Can you work these out from the model? Positions are in its coordinate system, mm. Face numbers are marked on the shaded views. A direction names the side the tool comes from. Coordinates: 2 decimals unless noted, no trailing zeros. Loops run counter-clockwise (first coordinate to the right, second up) from the corner with the lowest first, then second, coordinate; pieces in that order, holes last.
```python
from build123d import *

# Parameters (mm, degrees)
CYLINDER013_R     = 9.3
CYLINDER013_DEPTH = 30
BOX004_W          = 38
BOX004_H          = 16
BOX004_DEPTH      = 16
FILLET002_R       = 1
BOX003_W          = 20
BOX003_H          = 33
BOX003_DEPTH      = 16
FILLET001_R       = 1
BOX002_W          = 33
BOX002_H          = 27
BOX002_DEPTH      = 20
FILLET_R          = 2
CHAMFER003_SIZE   = 12
CHAMFER004_SIZE   = 18
CHAMFER005_SIZE   = 6.7
CHAMFER006_SIZE   = 6.8
CYLINDER012_R     = 9.3
CYLINDER012_DEPTH = 30
CYLINDER011_R     = 14
CYLINDER011_DEPTH = 15


with BuildPart() as cilindro013:
    # Cylinder013 → Cylinder013 (new body)
    with BuildSketch(Plane(origin=(27, 199, 74), x_dir=(1, 0, 0), z_dir=(0, -1, 0))):
        Circle(CYLINDER013_R)
    extrude(amount=CYLINDER013_DEPTH)


with BuildPart() as fillet002:
    # Box004 → Box004 (new body)
    with BuildSketch(Plane(origin=(-7, 189, 60), x_dir=(1, 0, 0), z_dir=(0, 0, 1))):
        with Locations((19, 8)):
            Rectangle(BOX004_W, BOX004_H)
    extrude(amount=BOX004_DEPTH)

    # Fillet002
    fillet002_edges = [fillet002.edges().sort_by_distance(p)[0] for p in [
        (12, 189, 60),
    ]]
    fillet(fillet002_edges, radius=FILLET002_R)


with BuildPart() as fillet001:
    # Box003 → Box003 (new body)
    with BuildSketch(Plane(origin=(-7, 172, 60), x_dir=(1, 0, 0), z_dir=(0, 0, 1))):
        with Locations((10, 16.5)):
            Rectangle(BOX003_W, BOX003_H)
    extrude(amount=BOX003_DEPTH)

    # Fillet001
    fillet001_edges = [fillet001.edges().sort_by_distance(p)[0] for p in [
        (13, 188.5, 60),
    ]]
    fillet(fillet001_edges, radius=FILLET001_R)


with BuildPart() as cut006:
    # Box002 → Box002 (new body)
    with BuildSketch(Plane(origin=(-5, 174, 53.3), x_dir=(1, 0, 0), z_dir=(0, 0, 1))):
        with Locations((16.5, 13.5)):
            Rectangle(BOX002_W, BOX002_H)
    extrude(amount=BOX002_DEPTH)

    # Fillet
    fillet_edges = [cut006.edges().sort_by_distance(p)[0] for p in [
        (-5, 201, 63.3),
    ]]
    fillet(fillet_edges, radius=FILLET_R)

    # Chamfer003
    chamfer003_edges = [cut006.edges().sort_by_distance(p)[0] for p in [
        (28, 201, 63.3),
    ]]
    chamfer(chamfer003_edges, length=CHAMFER003_SIZE)

    # Chamfer004
    chamfer004_edges = [cut006.edges().sort_by_distance(p)[0] for p in [
        (-5, 174, 63.3),
    ]]
    chamfer(chamfer004_edges, length=CHAMFER004_SIZE)

    # Chamfer005
    chamfer005_edges = [cut006.edges().sort_by_distance(p)[0] for p in [
        (20.5, 174, 53.3),
    ]]
    chamfer(chamfer005_edges, length=CHAMFER005_SIZE)

    # Chamfer006
    chamfer006_edges = [cut006.edges().sort_by_distance(p)[0] for p in [
        (28, 184.85, 53.3),
    ]]
    chamfer(chamfer006_edges, length=CHAMFER006_SIZE)

    # Cut004: cut Fillet001
    add(fillet001.part, mode=Mode.SUBTRACT)

    # Cut005: cut Fillet002
    add(fillet002.part, mode=Mode.SUBTRACT)

    # Cut006: cut Cilindro013
    add(cilindro013.part, mode=Mode.SUBTRACT)


with BuildPart() as cilindro012:
    # Cylinder012 → Cylinder012 (new body)
    with BuildSketch(Plane(origin=(27, 199, 74), x_dir=(1, 0, 0), z_dir=(0, -1, 0))):
        Circle(CYLINDER012_R)
    extrude(amount=CYLINDER012_DEPTH)


with BuildPart() as inductive_probe_mount:
    # Cylinder011 → Cylinder011 (new body)
    with BuildSketch(Plane(origin=(27, 189, 74), x_dir=(1, 0, 0), z_dir=(0, -1, 0))):
        Circle(CYLINDER011_R)
    extrude(amount=CYLINDER011_DEPTH)

    # Cut003: cut Cilindro012
    add(cilindro012.part, mode=Mode.SUBTRACT)

    # Fusion005: union Cut006
    add(cut006.part)


solid = inductive_probe_mount.part
```
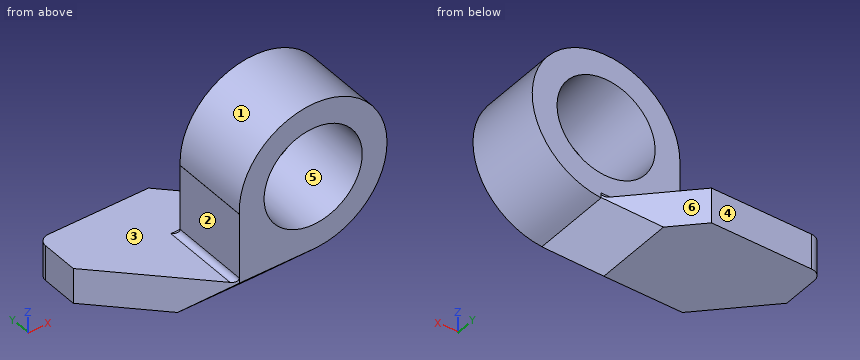
Item 1: Suppose I cut it at D-D, the plane z = 65.5. Please give me the cut outline in (x, y), plus the area to 3 significant figures.
Results are:
outline: (13, 174) - (23.23, 174) - (23.23, 189) - (13, 189) - close; (30.77, 174) - (38.12, 174) - (38.12, 189) - (30.77, 189) - close
area: 264 mm2
Item 2: I need wall thicknesses on line 1 along X through (y, z) = (178.25, 74); line 2 along Z through (x, y) = (27, 183); line 3 along X through (y, z) = (184.75, 69.5). Which ranges of each line are inside material? Lowest first, please.
Results are:
line 1: x = 13 to 17.7, 36.3 to 41
line 2: z = 59.1 to 64.7, 83.3 to 88
line 3: x = 13 to 18.86, 35.14 to 40.26
Item 3: I'm going to push flat-ended pins straight in: P1, Ø3, axis at y = 187.5, z = 66, coming from the +X side; P2, Ø6, axis at x = 17.5, y = 190.5, coming from the +Z side; P3, Ø10, axis at y = 178, z = 69, coming from the -X side. Where does each tip first touch, or does it pass through?
Results are:
P1: stops at x = 39.4
P2: stops at z = 86.18
P3: stops at x = 13
Item 4: We'd pull the mould along X, two halves only. Please class the marked faces 4, 5 and 6: +X half, -X half, draft (parallel to the pull), parting line (faces both ways), or undercut.
Results are:
face 4: draft
face 5: undercut
face 6: +X half
Item 5: Suppose I cut it at A-A, the plane z = 74. Please give me the cut outline in (x, y), plus the area to 3 significant figures.
Results are:
outline: (13, 174) - (17.7, 174) - (17.7, 189) - (13, 189) - close; (36.3, 174) - (41, 174) - (41, 189) - (36.3, 189) - close
area: 141 mm2
Item 6: Suppose I cut it at C-C, the plane x = 2.5. Please give me the cut outline in (y, z).
Results are:
outline: (184.5, 53.3) - (201, 53.3) - (201, 60) - (184.5, 60) - close
Item 7: On a 3-axis mill with a long thin cutter (end or side, diameter ignored), from which of +Z, -Z, +X, -X, +Y, -Y can I reach the whole of each face in a straight line? I mean the marked faces 1, 2 and 3. Say none if no direction works.
Results are:
face 1: +Y, -Y
face 2: +Z, -X, +Y, -Y
face 3: +Z, -X, +Y
